```python
from build123d import *

# Parameters (mm, degrees)
BOSS_EXTRUDE1_DEPTH = 2


with BuildPart() as part:
    # Sketch2 → Boss-Extrude1 (new body)
    with BuildSketch(Plane(origin=(0, 0, 0), x_dir=(1, 0, 0), z_dir=(0, 1, 0))):
        with BuildLine():
            Line((43.464851994, 1.5), (0.901387819, 1.5))
            ThreePointArc((0.901387819, 1.5), (1.523142916, 0.861705088), (1.75, 0))
            ThreePointArc((1.75, 0), (1.523142916, -0.861705088), (0.901387819, -1.5))
            Line((0.901387819, -1.5), (43.499845541, -1.5))
            ThreePointArc((43.499845541, -1.5), (42.633624493, -0.009899958), (43.464851994, 1.5))
        make_face()
        with BuildLine():
            Line((0.901387819, 1.5), (0, 1.5))
            Line((0, 1.5), (0, 1.25))
            ThreePointArc((0, 1.25), (0.883883476, 0.883883476), (1.25, 0))
            ThreePointArc((1.25, 0), (0.883883476, -0.883883476), (0, -1.25))
            Line((0, -1.25), (0, -1.5))
            Line((0, -1.5), (0.901387819, -1.5))
            ThreePointArc((0.901387819, -1.5), (1.523142916, -0.861705088), (1.75, 0))
            ThreePointArc((1.75, 0), (1.523142916, 0.861705088), (0.901387819, 1.5))
        make_face()
        with BuildLine():
            Line((0, 1.5), (0, 1.75))
            ThreePointArc((0, 1.75), (-1.75, 0), (0, -1.75))
            Line((0, -1.75), (0, -1.5))
            Line((0, -1.5), (0, -1.25))
            ThreePointArc((0, -1.25), (-1.25, 0), (0, 1.25))
            Line((0, 1.25), (0, 1.5))
        make_face()
        with BuildLine():
            Line((44.383505452, 1.760511556), (44.383505452, 1.5))
            Line((44.383505452, 1.5), (44.383505452, 1.239488444))
            ThreePointArc((44.383505452, 1.239488444), (45.267388929, 0.87337192), (45.633505452, -0.010511556))
            ThreePointArc((45.633505452, -0.010511556), (45.267388929, -0.894395033), (44.383505452, -1.260511556))
            Line((44.383505452, -1.260511556), (44.383505452, -1.5))
            Line((44.383505452, -1.5), (44.383505452, -1.739488444))
            ThreePointArc((44.383505452, -1.739488444), (45.620942319, -1.226925311), (46.133505452, 0.010511556))
            ThreePointArc((46.133505452, 0.010511556), (45.620942319, 1.247948423), (44.383505452, 1.760511556))
        make_face()
        with BuildLine():
            Line((44.383505452, 1.5), (43.464851994, 1.5))
            ThreePointArc((43.464851994, 1.5), (42.633624493, -0.009899958), (43.499845541, -1.5))
            Line((43.499845541, -1.5), (44.383505452, -1.5))
            Line((44.383505452, -1.5), (44.383505452, -1.260511556))
            ThreePointArc((44.383505452, -1.260511556), (43.133505452, -0.010511556), (44.383505452, 1.239488444))
            Line((44.383505452, 1.239488444), (44.383505452, 1.5))
        make_face()
        with BuildLine():
            ThreePointArc((0.901387819, 1.5), (0.467707173, 1.686342195), (0, 1.75))
            Line((0, 1.75), (0, 1.5))
            Line((0, 1.5), (0.901387819, 1.5))
        make_face()
        with BuildLine():
            Line((0, -1.5), (0, -1.75))
            ThreePointArc((0, -1.75), (0.467707173, -1.686342195), (0.901387819, -1.5))
            Line((0.901387819, -1.5), (0, -1.5))
        make_face()
        with BuildLine():
            ThreePointArc((44.383505452, 1.760511556), (43.906066857, 1.694124454), (43.464851994, 1.5))
            Line((43.464851994, 1.5), (44.383505452, 1.5))
            Line((44.383505452, 1.5), (44.383505452, 1.760511556))
        make_face()
        with BuildLine():
            Line((44.383505452, -1.5), (43.499845541, -1.5))
            ThreePointArc((43.499845541, -1.5), (43.925736528, -1.678555527), (44.383505452, -1.739488444))
            Line((44.383505452, -1.739488444), (44.383505452, -1.5))
        make_face()
    extrude(amount=BOSS_EXTRUDE1_DEPTH)


solid = part.part
```
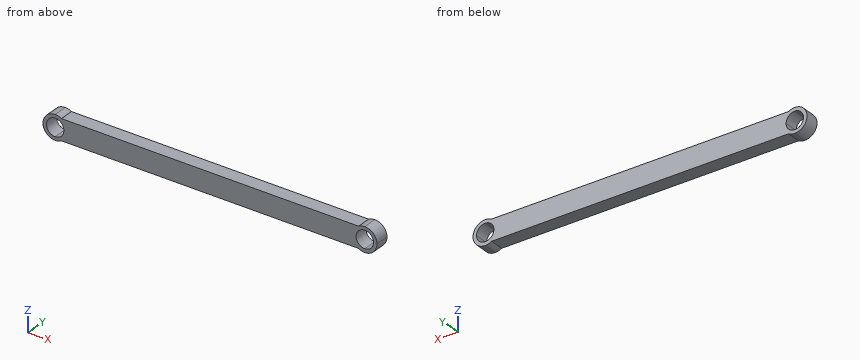
Part model, mm, in its own coordinate system. Round coordinates to 2 decimals unless told otherwise and drop trailing zeros. Write each loop counter-clockwise with the first axis right and the second up, starting at its lowest first coordinate (ties: lowest second). Pieces come first, ordered by that corner, then holes. Notation, with made-up numbers: (44, 79.25) -> (49, 79.25) arc R20 ccw to (49, 109.25) -> close; hole circle Ø10 at (-1.75, 45.25). An arc over 180 degrees is marked (long way). Return JSON: item names as keys, results as strings. Group by question number.
Q1. Saw through at B-B on x = 34. Write the cut outline in (y, z), plus the area to 3 significant figures.
Q2. Saw through at A-A on y = 1.25. Write the cut outline in (x, z), plus the area to 3 significant figures.
Q3. Pin check, flat tip, straight feed: pin 1 (1 mm diameter, centred on x = 15.5, y = 1, fed in from -Z). Stop position of the tip, or through.
Q4. Probe L1, parallel to X at y = 1.6, z = 0.4; L2, parallel to X at y = 0.2, z = 0.55; L3, parallel to Z at x = 6.5, y = 0.25. List the from-to ranges inside material, lowest first. Write a range as [from, to].
Answer:
{
 "1": {"outline": "(0, -1.5) -> (2, -1.5) -> (2, 1.5) -> (0, 1.5) -> close", "area": "6.00 mm2"},
 "2": {"outline": "(0.9, -1.5) -> (43.46, -1.5) arc R1.75 ccw (long way) to (43.5, 1.5) -> (0.9, 1.5) arc R1.75 ccw (long way) to start; hole circle Ø2.5 at (0, 0); hole circle Ø2.5 at (44.38, 0.01)", "area": "134 mm2"},
 "3": {"pin 1": "z = -1.5"},
 "4": {"L1": "[-1.7, -1.18], [1.18, 43.2], [45.57, 46.08]", "L2": "[-1.66, -1.12], [1.12, 43.26], [45.51, 46.04]", "L3": "[-1.5, 1.5]"}
}
